Check sheet for the drawn part. Datum: minimum x, y, z corner. Units: mm. Round coordinates to 2 decimals unless told otherwise and drop trailing zeros. Order: outer loops, then holes, each group sorted by start corner. A loop starts at its lowest first (then second) coordinate and runs counter-clockwise, first axis right, second up. Notation, with made-up numbers: (81, -32.75) -> (134, -32.75) arc R12 ccw to (134, -18.75) -> close; hole circle Ø5 at (34.25, -30). An arc over 180 degrees is marked (long way). Use CSV: the item, a comma, the result in double quotes.
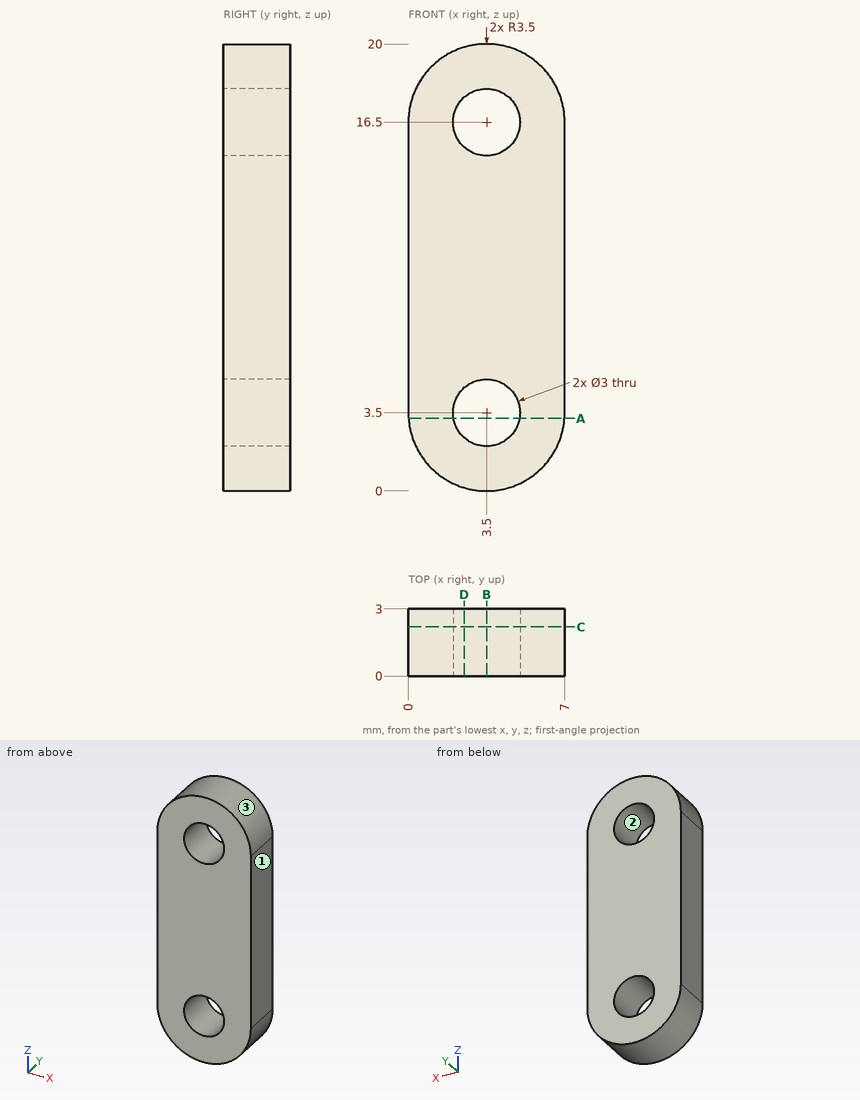
Q1. Go/stop test with flat-tipped pins: pin 1 (1 mm diameter, centred on y = 1.5, z = 17.5, fed in from +X); pin 2 (1.5 mm diameter, centred on x = 4.5, y = 2, fed in from +Z). Record where each tip stops, or that it passes through.
Result sheet:
pin 1,"stops at x = 6.96"
pin 2,"stops at z = 19.99"
Q2. Sectioned sample at C-C, the plane y = 2.2. Enter the section's corners in (x, z), then the cut area to 3 significant figures.
Result sheet:
outline,"(0, 3.5) arc R3.5 ccw to (7, 3.5) -> (7, 16.5) arc R3.5 ccw to (0, 16.5) -> close; hole circle Ø3 at (3.5, 3.5); hole circle Ø3 at (3.5, 16.5)"
area,"115 mm^2"
Q3. Scan lines: L1, parallel to Z at x = 3.5, y = 0.9; L2, parallel to Z at x = 4.5, y = 2.6; L3, parallel to X at y = 2.55, z = 3.5. Record each from-to range of solid material in increasing order.
Result sheet:
L1,"z = 0 to 2, 5 to 15, 18 to 20"
L2,"z = 0.15 to 2.38, 4.62 to 15.38, 17.62 to 19.85"
L3,"x = 0 to 2, 5 to 7"
Q4. Mould release check, pull along X, two halves, no side actions. Record for the marked faces 1, 2 and 3: pulls with the +X half, pulls with the -X half, needs draft (parallel to the pull), parting line crosses it, or undercut.
Result sheet:
face 1,"pulls with the +X half"
face 2,"undercut"
face 3,"parting line crosses it"
Q5. Sectioned sample at A-A, the plane z = 3.25. Enter the section's corners in (x, y), then the cut area to 3 significant figures.
Result sheet:
outline,"(0.01, 0) -> (2.02, 0) -> (2.02, 3) -> (0.01, 3) -> close; (4.98, 0) -> (6.99, 0) -> (6.99, 3) -> (4.98, 3) -> close"
area,"12.1 mm^2"
Q6. Sectioned sample at D-D, the plane x = 2.5. Enter the section's corners in (y, z).
Result sheet:
outline,"(0, 0.15) -> (3, 0.15) -> (3, 2.38) -> (0, 2.38) -> close; (0, 4.62) -> (3, 4.62) -> (3, 15.38) -> (0, 15.38) -> close; (0, 17.62) -> (3, 17.62) -> (3, 19.85) -> (0, 19.85) -> close"
Q7. Sectioned sample at B-B, the plane x = 3.5. Enter the section's corners in (y, z).
Result sheet:
outline,"(0, 0) -> (3, 0) -> (3, 2) -> (0, 2) -> close; (0, 5) -> (3, 5) -> (3, 15) -> (0, 15) -> close; (0, 18) -> (3, 18) -> (3, 20) -> (0, 20) -> close"
